```python
from build123d import *

# Parameters (mm, degrees)
SKETCH1_W           = 576.6975777
SKETCH1_H           = 526.6975777
SKETCH1_R           = 2.5
BOSS_EXTRUDE1_DEPTH = 5
SKETCH2_R           = 10
CUT_EXTRUDE1_DEPTH  = 10


with BuildPart() as part:
    # Sketch1 → Boss-Extrude1 (new body)
    with BuildSketch(Plane.XY):
        with Locations((288.34878885, 263.34878885)):
            Rectangle(SKETCH1_W, SKETCH1_H)
        with Locations((7.644193715, 265.84878885)):
            Circle(SKETCH1_R, mode=Mode.SUBTRACT)
        with Locations((569.053383985, 265.84878885)):
            Circle(SKETCH1_R, mode=Mode.SUBTRACT)
    extrude(amount=BOSS_EXTRUDE1_DEPTH)

    # Sketch2 → Cut-Extrude1 (cut)
    with BuildSketch(Plane(origin=(0, 0, 0), x_dir=(-1, 0, 0), z_dir=(0, 0, -1))):
        with Locations((-288.34878885, 50)):
            Circle(SKETCH2_R)
    extrude(amount=-CUT_EXTRUDE1_DEPTH, mode=Mode.SUBTRACT)


solid = part.part
```
Read the model definition and answer for the solid it produces. Units are mm, in the model's axes. Round coordinates to 2 decimals unless told otherwise and drop trailing zeros. Write each loop counter-clockwise with the first axis right and the second up, starting at its lowest first coordinate (ties: lowest second). Pieces come first, ordered by that corner, then holes. Notation, with made-up numbers: (-10.75, -37.75) - (1.25, -37.75) arc R22 ccw to (1.25, -9.75) - close; hole circle Ø3 at (66, 76). An arc over 180 degrees is marked (long way). One line per item, written item: value.
Q1. Find section A-A (y = 50). Determine the outline of the cut face in (x, z), and give its area (3 significant figures).
The answers:
outline: (0, 0) - (278.35, 0) - (278.35, 5) - (0, 5) - close; (298.35, 0) - (576.7, 0) - (576.7, 5) - (298.35, 5) - close
area: 2,780 mm2
Q2. For a pull along Y with two mould halves and no side action, classify faces 1 (the flat face through (284, 267, 5)), 2 (the cylindrical face through (279.1, 46.2, 2.5)) as pulls with the +Y half, pulls with the -Y half, needs draft (parallel to the pull), parting line crosses it, or undercut.
The answers:
face 1: needs draft
face 2: undercut
Q3. Straight lines are drawn through the part: line 1 (Y direction, x = 282.5, z = 1.1); line 2 (Y direction, x = 285.5, z = 2.75). For each, find the intervals that lie inside material, in ascending order. Write a range as from..to.
The answers:
line 1: y = 0..41.89, 58.11..526.7
line 2: y = 0..40.41, 59.59..526.7
